```python
from build123d import *

# Parameters (mm, degrees)
BOSS_EXTRUDE1_DEPTH      = 20.5
SHELL1_START             = -12.7000001
SHELL1_OUTLINE_W         = 39
SHELL1_OUTLINE_H         = 35.5
SHELL1_DEPTH             = 35.7000001
SKETCH27_R               = 0.5
CUT_EXTRUDE10_DEPTH      = 1
CUT_EXTRUDE17_DEPTH      = 40.36051338
CUT_EXTRUDE17_DEPTH_BACK = 40.36051338
SKETCH35_R               = 4.25


# Read off the part's stored shape, not the designer's step: Shell1, CBORE for M2 Hex Socket Head Cap Screw2
with BuildPart() as part:
    # Sketch4 → Boss-Extrude1 (new, symmetric)
    with BuildSketch(Plane.XY):
        with BuildLine():
            Line((27, -18), (27, 20))
            add(Edge.make_bspline(
                [(-7.730668476, 10.076049072), (2.170162487, 17.672284588), (21.370784375, 20), (27, 20)],
                knots=[0, 0, 0, 0, 1, 1, 1, 1], degree=3))
            ThreePointArc((-7.730668476, 10.076049072), (-12.308703382, -3.128229699), (-1.981723336, -12.544431937))
            add(Edge.make_bspline(
                [(-1.981723336, -12.544431937), (7.580415063, -14.055023481), (14.656713895, -12.657176609), (27, -18)],
                knots=[0, 0, 0, 0, 1, 1, 1, 1], degree=3))
        make_face()
    extrude(amount=BOSS_EXTRUDE1_DEPTH, both=True)

    # Shell1 outline → Shell1 (cut)
    with BuildSketch(Plane.YZ.offset(SHELL1_START)):
        with Locations((1.5, 0)):
            Rectangle(SHELL1_OUTLINE_W, SHELL1_OUTLINE_H)
    extrude(amount=SHELL1_DEPTH, mode=Mode.SUBTRACT)

    # CBORE for M2 Hex Socket Head Cap Scr 2 → CBORE for M2 Hex Socket Head Cap Screw2 (revolve, cut)
    with BuildSketch(Plane(origin=(-5.656854249, -5.656854249, 0), x_dir=(1, 0, 0), z_dir=(0, -1, 0))):
        Polygon((0, 17.75), (1.15, 17.75), (1.15, 19), (1.2, 19.05), (2.3, 19.05), (2.3, 20.5), (0, 20.5), align=None)
    cbore_for_m2_hex_socket_head_cap_screw2 = revolve(axis=Axis((-5.656854249, -5.656854249, 0), (0, 0, 1)), mode=Mode.SUBTRACT)

    # CBORE for M2 Hex Socket Head Cap Scr 3 o → CBORE for M2 Hex Socket Head Cap Scr 3 (revolve, cut)
    with BuildSketch(Plane(origin=(-8, 0, 0), x_dir=(1, 0, 0), z_dir=(0, -1, 0))):
        Polygon((1.15, 19), (1.2, 19.05), (2.3, 19.05), (2.3, 20.5), (0, 20.5), (0, 17.75), (1.15, 17.75), align=None)
    cbore_for_m2_hex_socket_head_cap_scr_3 = revolve(axis=Axis((-8, 0, 0), (0, 0, 1)), mode=Mode.SUBTRACT)

    # CBORE for M2 Hex Socket Head Cap Scr 4 o → CBORE for M2 Hex Socket Head Cap Scr 4 (revolve, cut)
    with BuildSketch(Plane(origin=(-5.656854249, 5.656854249, 0), x_dir=(1, 0, 0), z_dir=(0, -1, 0))):
        Polygon((1.15, 19), (1.2, 19.05), (2.3, 19.05), (2.3, 20.5), (0, 20.5), (0, 17.75), (1.15, 17.75), align=None)
    cbore_for_m2_hex_socket_head_cap_scr_4 = revolve(axis=Axis((-5.656854249, 5.656854249, 0), (0, 0, 1)), mode=Mode.SUBTRACT)

    # CBORE for M2 Hex Socket Head Cap Scr 5 o → CBORE for M2 Hex Socket Head Cap Scr 5 (revolve, cut)
    with BuildSketch(Plane(origin=(8, 0, 0), x_dir=(1, 0, 0), z_dir=(0, -1, 0))):
        Polygon((1.15, 19), (1.2, 19.05), (2.3, 19.05), (2.3, 20.5), (0, 20.5), (0, 17.75), (1.15, 17.75), align=None)
    cbore_for_m2_hex_socket_head_cap_scr_5 = revolve(axis=Axis((8, 0, 0), (0, 0, 1)), mode=Mode.SUBTRACT)

    # CBORE for M2 Hex Socket Head Cap Scr 6 o → CBORE for M2 Hex Socket Head Cap Scr 6 (revolve, cut)
    with BuildSketch(Plane(origin=(5.656854249, -5.656854249, 0), x_dir=(1, 0, 0), z_dir=(0, -1, 0))):
        Polygon((1.15, 19), (1.2, 19.05), (2.3, 19.05), (2.3, 20.5), (0, 20.5), (0, 17.75), (1.15, 17.75), align=None)
    cbore_for_m2_hex_socket_head_cap_scr_6 = revolve(axis=Axis((5.656854249, -5.656854249, 0), (0, 0, 1)), mode=Mode.SUBTRACT)

    # CBORE for M2 Hex Socket Head Cap Scr 7 o → CBORE for M2 Hex Socket Head Cap Scr 7 (revolve, cut)
    with BuildSketch(Plane.XZ.offset(8)):
        Polygon((1.15, 19), (1.2, 19.05), (2.3, 19.05), (2.3, 20.5), (0, 20.5), (0, 17.75), (1.15, 17.75), align=None)
    cbore_for_m2_hex_socket_head_cap_scr_7 = revolve(axis=Axis((0, -8, 0), (0, 0, 1)), mode=Mode.SUBTRACT)

    # CBORE for M2 Hex Socket Head Cap Scr 8 o → CBORE for M2 Hex Socket Head Cap Scr 8 (revolve, cut)
    with BuildSketch(Plane.XZ.offset(-8)):
        Polygon((1.15, 19), (1.2, 19.05), (2.3, 19.05), (2.3, 20.5), (0, 20.5), (0, 17.75), (1.15, 17.75), align=None)
    cbore_for_m2_hex_socket_head_cap_scr_8 = revolve(axis=Axis((0, 8, 0), (0, 0, 1)), mode=Mode.SUBTRACT)

    # CBORE for M2 Hex Socket Head Cap Scr 9 o → CBORE for M2 Hex Socket Head Cap Scr 9 (revolve, cut)
    with BuildSketch(Plane(origin=(5.656854249, 5.656854249, 0), x_dir=(1, 0, 0), z_dir=(0, -1, 0))):
        Polygon((1.15, 19), (1.2, 19.05), (2.3, 19.05), (2.3, 20.5), (0, 20.5), (0, 17.75), (1.15, 17.75), align=None)
    cbore_for_m2_hex_socket_head_cap_scr_9 = revolve(axis=Axis((5.656854249, 5.656854249, 0), (0, 0, 1)), mode=Mode.SUBTRACT)

    # Sketch27 → Cut-Extrude10 (cut)
    with BuildSketch(Plane.XY.offset(20.5)):
        with Locations((-4.330127019, -2.5)):
            Circle(SKETCH27_R)
        with Locations((-4.330127019, 2.5)):
            Circle(SKETCH27_R)
        with Locations((5, 0)):
            Circle(SKETCH27_R)
    extrude(amount=-CUT_EXTRUDE10_DEPTH, mode=Mode.SUBTRACT)

    # Mirror2: CBORE for M2 Hex Socket Head Cap Screw2, CBORE for M2 Hex Socket Head Cap Scr 3, CBORE for M2 Hex Socket Head Cap Scr 4, CBORE for M2 Hex Socket Head Cap Scr 5, CBORE for M2 Hex Socket Head Cap Scr 6, CBORE for M2 Hex Socket Head Cap Scr 7, CBORE for M2 Hex Socket Head Cap Scr 8, CBORE for M2 Hex Socket Head Cap Scr 9 across plane
    add(cbore_for_m2_hex_socket_head_cap_screw2.mirror(Plane.XY), mode=Mode.SUBTRACT)
    add(cbore_for_m2_hex_socket_head_cap_scr_3.mirror(Plane.XY), mode=Mode.SUBTRACT)
    add(cbore_for_m2_hex_socket_head_cap_scr_4.mirror(Plane.XY), mode=Mode.SUBTRACT)
    add(cbore_for_m2_hex_socket_head_cap_scr_5.mirror(Plane.XY), mode=Mode.SUBTRACT)
    add(cbore_for_m2_hex_socket_head_cap_scr_6.mirror(Plane.XY), mode=Mode.SUBTRACT)
    add(cbore_for_m2_hex_socket_head_cap_scr_7.mirror(Plane.XY), mode=Mode.SUBTRACT)
    add(cbore_for_m2_hex_socket_head_cap_scr_8.mirror(Plane.XY), mode=Mode.SUBTRACT)
    add(cbore_for_m2_hex_socket_head_cap_scr_9.mirror(Plane.XY), mode=Mode.SUBTRACT)

    # Sketch35 → Cut-Extrude17 (cut, two sides: drawn at the far end of the back side and taken through both)
    with BuildSketch(Plane.XY.offset(-CUT_EXTRUDE17_DEPTH_BACK)):
        Circle(SKETCH35_R)
    extrude(amount=CUT_EXTRUDE17_DEPTH + CUT_EXTRUDE17_DEPTH_BACK, mode=Mode.SUBTRACT)


solid = part.part
```
Here's how the part is built. I have some questions about the finished solid (model axes, mm). A direction names the side the tool comes from. Coordinates: 2 decimals unless noted, no trailing zeros.
1) Imagine slicing it at A-A on x = 0. State how many separate pieces and enclosed holes the cut face has, and give its area (3 significant figures).
2) I need wall thicknesses on line 1 (Z direction, x = 13.5, y = 7); line 2 (Z direction, x = -1.5, y = 7); line 3 (X direction, y = 16, z = -17.5). Which ranges of each line are inside material? Lowest first, please.
3) Which directions (+Z, -Z, +X, -X, +Y, -Y) give clear straight access to the entire face, cutting with the end or side of a thin tool? Please do faces 1 (the face through (4.7, 4.7, -19.05)), 2 (the face through (4.7, 4.7, 19.05)), 3 (the face through (4.809, 6.434, 18.384)).
4) Will these pins go through, and if not, where does the flat tip stop? pin 1 (1.5 mm diameter, centred on y = -11, z = 0.5, fed in from -X); pin 2 (12 mm diameter, centred on x = 14, z = -12, fed in from +Y); pin 3 (1.4 mm diameter, centred on x = 4.5, y = 5.5, fed in from +Z).
Response values:
1. separate pieces: 8
1. enclosed holes: 0
1. area: 64.3 mm2
2. line 1: z = -20.5 to -17.75, 17.75 to 20.5
2. line 2: z = -19.05 to -17.75, 17.75 to 19.05
2. line 3: x = 23 to 27
3. face 1: -Z
3. face 2: +Z
3. face 3: +Z, -Z
4. pin 1: stops at x = 23
4. pin 2: stops at y = 18.79
4. pin 3: stops at z = 19.05
